from build123d import *

# Parameters (mm, degrees)
SKETCH_1_R      = 11
SKETCH_1_R_2    = 2.5
EXTRUDE_1_DEPTH = 2
SKETCH_2_R      = 9
SKETCH_2_R_2    = 2.5
EXTRUDE_2_DEPTH = 11
SKETCH_3_R      = 11
SKETCH_3_R_2    = 2.5
EXTRUDE_3_DEPTH = 2


with BuildPart() as part:
    # 草图1 → 凸台-拉伸1 (new body)
    with BuildSketch(Plane(origin=(0, 0, 0), x_dir=(0, 0, -1), z_dir=(1, 0, 0))):
        Circle(SKETCH_1_R)
        Circle(SKETCH_1_R_2, mode=Mode.SUBTRACT)
    extrude(amount=EXTRUDE_1_DEPTH)

    # 草图2 → 凸台-拉伸2 (add)
    with BuildSketch(Plane(origin=(2, 0, 0), x_dir=(0, 0, -1), z_dir=(1, 0, 0))):
        Circle(SKETCH_2_R)
        Circle(SKETCH_2_R_2, mode=Mode.SUBTRACT)
    extrude(amount=EXTRUDE_2_DEPTH)

    # 草图3 → 凸台-拉伸3 (add)
    with BuildSketch(Plane(origin=(13, 0, 0), x_dir=(0, 0, -1), z_dir=(1, 0, 0))):
        Circle(SKETCH_3_R)
        Circle(SKETCH_3_R_2, mode=Mode.SUBTRACT)
    extrude(amount=EXTRUDE_3_DEPTH)


solid = part.part
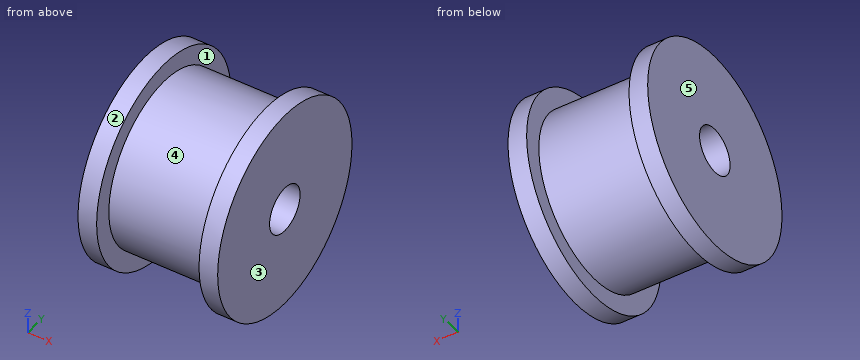
Verification items for the finished model (mm, model axes). Face numbers are marked on the shaded views. A direction names the side the tool comes from. Coordinates: 2 decimals unless noted, no trailing zeros. Loops run counter-clockwise (first coordinate to the right, second up) from the corner with the lowest first, then second, coordinate; pieces in that order, holes last. Notation, with made-up numbers: M 49.5,81.5 L 101.5,81.5 A21 cw 101.5,90.5 Z; hole C -15.75,21 d4. An arc over 180 degrees is marked long. One line per item, written item: value.
1. Section check D-D on y = -4.75. Record the cut outline in (x, z).
Answers follow:
outline: M 0,-9.92 L 2,-9.92 L 2,-7.64 L 13,-7.64 L 13,-9.92 L 15,-9.92 L 15,9.92 L 13,9.92 L 13,7.64 L 2,7.64 L 2,9.92 L 0,9.92 Z
2. Mould release check, pull along X, two halves, no side actions. Record for the marked faces 1, 2 and 3: pulls with the +X half, pulls with the -X half, needs draft (parallel to the pull), parting line crosses it, or undercut.
Answers follow:
face 1: undercut
face 2: needs draft
face 3: pulls with the +X half
3. Section check A-A on y = 0. Record the cut outline in (x, z), plus the area to 3 significant figures.
Answers follow:
outline: M 0,-11 L 2,-11 L 2,-9 L 13,-9 L 13,-11 L 15,-11 L 15,-2.5 L 0,-2.5 Z; M 0,2.5 L 15,2.5 L 15,11 L 13,11 L 13,9 L 2,9 L 2,11 L 0,11 Z
area: 211 mm^2
4. Section check C-C on x = 1.5. Record the cut outline in (y, z), plus the area to 3 significant figures.
Answers follow:
outline: C 0,0 d22; hole C 0,0 d5
area: 360 mm^2
5. Set-up check for the marked faces 4 and 5: record each of +Z, -Z, +X, -X, +Y, -Y from which the full face is reachable in a straight line by a thin tool's end or side.
Answers follow:
face 4: none
face 5: +Z, -Z, -X, +Y, -Y
6. Gauge pin test, flat ends, axial feed: P1, Ø1.5, axis at x = 5, z = -3, coming from the +Y side; P2, Ø4.5, axis at y = 0, z = 0, coming from the +X side; P3, Ø4, axis at x = 7.5, z = 0, coming from the -Y side; P4, Ø4, axis at x = 13.5, z = -6, coming from the -Y side. Record the tip position at first contact, or that the pin passes through.
Answers follow:
P1: y = 8.71
P2: through
P3: y = -9
P4: y = -10.25
7. Material ranges on line 1 along Y through (x, z) = (9.5, 0); line 2 along X through (y, z) = (9.25, 1); line 3 along Y through (x, z) = (10.25, 8), recorded low to high. Write a range as from..to.
Answers follow:
line 1: -9..-2.5, 2.5..9
line 2: 0..2, 13..15
line 3: -4.12..4.12
